from build123d import *
from OCP.BRepFilletAPI import BRepFilletAPI_MakeChamfer
from build123d.topology import SkipClean

# Parameters (mm, degrees)
SKETCH2_R           = 40
SKETCH2_R_2         = 20
BOSS_EXTRUDE1_DEPTH = 8
BOSS_EXTRUDE2_DEPTH = 12
SKETCH4_R           = 7.5
CUT_EXTRUDE1_DEPTH  = 10
SKETCH5_R           = 4
CUT_EXTRUDE2_DEPTH  = 29
BOSS_EXTRUDE3_DEPTH = 8
CHAMFER3_SIZE       = 8
CHAMFER3_SIZE_2     = 19.800694827
BOSS_EXTRUDE4_DEPTH = 12
FILLET1_R           = 6
CUT_EXTRUDE3_DEPTH  = 6
SKETCH9_R           = 4.2
CUT_EXTRUDE4_DEPTH  = 6
CUT_EXTRUDE5_START  = -22
CUT_EXTRUDE5_DEPTH  = 22


with BuildPart() as part:
    # Sketch2 → Boss-Extrude1 (new body)
    with BuildSketch(Plane.XY):
        Circle(SKETCH2_R)
        Circle(SKETCH2_R_2, mode=Mode.SUBTRACT)
    extrude(amount=BOSS_EXTRUDE1_DEPTH)

    # Sketch3 → Boss-Extrude2 (add)
    with BuildSketch(Plane(origin=(0, 0, 0), x_dir=(-1, 0, 0), z_dir=(0, 0, -1))):
        with BuildLine():
            Line((105, -25), (105, 25))
            Line((105, 25), (20.894189842, 56.244402662))
            ThreePointArc((20.894189842, 56.244402662), (-60, 0), (20.894189842, -56.244402662))
            Line((20.894189842, -56.244402662), (105, -25))
        make_face()
    extrude(amount=BOSS_EXTRUDE2_DEPTH)

    # Sketch4 → Cut-Extrude1 (cut)
    with BuildSketch(Plane(origin=(0, 0, -12), x_dir=(-1, 0, 0), z_dir=(0, 0, -1))):
        with Locations((0, 30)):
            Circle(SKETCH4_R)
        with Locations((30, 0)):
            Circle(SKETCH4_R)
        with Locations((0, -30)):
            Circle(SKETCH4_R)
        with Locations((-30, 0)):
            Circle(SKETCH4_R)
    extrude(amount=-CUT_EXTRUDE1_DEPTH, mode=Mode.SUBTRACT)

    # Sketch5 → Cut-Extrude2 (cut)
    with BuildSketch(Plane(origin=(0, 0, -2), x_dir=(-1, 0, 0), z_dir=(0, 0, -1))):
        with Locations((30, 0)):
            Circle(SKETCH5_R)
        with Locations((0, -30)):
            Circle(SKETCH5_R)
        with Locations((-30, 0)):
            Circle(SKETCH5_R)
        with Locations((0, 30)):
            Circle(SKETCH5_R)
    extrude(amount=-CUT_EXTRUDE2_DEPTH, mode=Mode.SUBTRACT)

    # Sketch6 → Boss-Extrude3 (add)
    with SkipClean():  # the faces are left unmerged after this step: merging them gives an invalid solid
        with BuildSketch(Plane.XY):
            with BuildLine():
                Line((39.290584114, -7.5), (59.529404499, -7.5))
                ThreePointArc((59.529404499, -7.5), (60, 0), (59.529404499, 7.5))
                Line((59.529404499, 7.5), (39.290584114, 7.5))
                ThreePointArc((39.290584114, 7.5), (40, 0), (39.290584114, -7.5))
            make_face()
            with BuildLine():
                Line((-7.5, 39.290584114), (-7.5, 59.529404499))
                ThreePointArc((-7.5, 59.529404499), (0, 60), (7.5, 59.529404499))
                Line((7.5, 59.529404499), (7.5, 39.290584114))
                ThreePointArc((7.5, 39.290584114), (0, 40), (-7.5, 39.290584114))
            make_face()
            with BuildLine():
                Line((-7.5, -39.290584114), (-7.5, -59.529404499))
                ThreePointArc((-7.5, -59.529404499), (0, -60), (7.5, -59.529404499))
                Line((7.5, -59.529404499), (7.5, -39.290584114))
                ThreePointArc((7.5, -39.290584114), (0, -40), (-7.5, -39.290584114))
            make_face()
            with BuildLine():
                Line((-39.290584114, 7.5), (-59.529404499, 7.5))
                ThreePointArc((-59.529404499, 7.5), (-60, 0), (-59.529404499, -7.5))
                Line((-59.529404499, -7.5), (-39.290584114, -7.5))
                ThreePointArc((-39.290584114, -7.5), (-40, 0), (-39.290584114, 7.5))
            make_face()
        extrude(amount=BOSS_EXTRUDE3_DEPTH)

    # Chamfer3
    chamfer3_edges_1 = [part.edges().sort_by_distance(p)[0] for p in [
        (0, 60, 8),
    ]]
    chamfer3_side_1 = [part.faces().sort_by_distance(p)[0] for p in [
        (0, 60, 7.84),
    ]]
    chamfer3_edges_2 = [part.edges().sort_by_distance(p)[0] for p in [
        (60, 0, 8),
    ]]
    chamfer3_side_2 = [part.faces().sort_by_distance(p)[0] for p in [
        (60, 0, 7.84),
    ]]
    chamfer3_edges_3 = [part.edges().sort_by_distance(p)[0] for p in [
        (-60, 0, 8),
    ]]
    chamfer3_side_3 = [part.faces().sort_by_distance(p)[0] for p in [
        (-60, 0, 7.84),
    ]]
    chamfer3_edges_4 = [part.edges().sort_by_distance(p)[0] for p in [
        (0, -60, 8),
    ]]
    chamfer3_side_4 = [part.faces().sort_by_distance(p)[0] for p in [
        (0, -60, 7.84),
    ]]
    chamfer3 = BRepFilletAPI_MakeChamfer(part.part.solid().wrapped)
    for e in chamfer3_edges_1:
        chamfer3.Add(CHAMFER3_SIZE - 0.0001, CHAMFER3_SIZE_2 - 0.0001, e.wrapped, chamfer3_side_1[0].wrapped)
    for e in chamfer3_edges_2:
        chamfer3.Add(CHAMFER3_SIZE - 0.0001, CHAMFER3_SIZE_2 - 0.0001, e.wrapped, chamfer3_side_2[0].wrapped)
    for e in chamfer3_edges_3:
        chamfer3.Add(CHAMFER3_SIZE - 0.0001, CHAMFER3_SIZE_2 - 0.0001, e.wrapped, chamfer3_side_3[0].wrapped)
    for e in chamfer3_edges_4:
        chamfer3.Add(CHAMFER3_SIZE - 0.0001, CHAMFER3_SIZE_2 - 0.0001, e.wrapped, chamfer3_side_4[0].wrapped)
    add(Compound.cast(chamfer3.Shape()), mode=Mode.REPLACE)  # a hair under: the kernel refuses the full size

    # Sketch7 → Boss-Extrude4 (add)
    with BuildSketch(Plane(origin=(0, 0, -12), x_dir=(-1, 0, 0), z_dir=(0, 0, -1))):
        with BuildLine():
            Line((115, 12.5), (105, 12.5))
            Line((105, 12.5), (105, -12.5))
            Line((105, -12.5), (115, -12.5))
            ThreePointArc((115, -12.5), (127.5, 0), (115, 12.5))
        make_face()
    extrude(amount=-BOSS_EXTRUDE4_DEPTH)

    # Fillet1
    fillet1_edges = [part.edges().sort_by_distance(p)[0] for p in [
        (-105, -25, -6),
        (-105, 25, -6),
        (-105, -12.5, -6),
        (-105, 12.5, -6),
    ]]
    fillet(fillet1_edges, radius=FILLET1_R)

    # Sketch8 → Cut-Extrude3 (cut)
    with SkipClean():  # the faces are left unmerged after this step: merging them gives an invalid solid
        with BuildSketch(Plane(origin=(0, 0, -12), x_dir=(-1, 0, 0), z_dir=(0, 0, -1))):
            Polygon((118.778590974, 6.485027647), (111.2730968, 6.514869597), (107.494505826, 0.02984195), (111.221409026, -6.485027647), (118.7269032, -6.514869597), (122.505494174, -0.02984195), align=None)
        extrude(amount=-CUT_EXTRUDE3_DEPTH, mode=Mode.SUBTRACT)

    # Sketch9 → Cut-Extrude4 (cut)
    with SkipClean():  # the faces are left unmerged after this step: merging them gives an invalid solid
        with BuildSketch(Plane(origin=(0, 0, -6), x_dir=(-1, 0, 0), z_dir=(0, 0, -1))):
            with Locations((115, 0)):
                Circle(SKETCH9_R)
        extrude(amount=-CUT_EXTRUDE4_DEPTH, mode=Mode.SUBTRACT)

    # Sketch10 → Cut-Extrude5 (cut)
    with SkipClean():  # the faces are left unmerged after this step: merging them gives an invalid solid
        with BuildSketch(Plane.XY.offset(CUT_EXTRUDE5_START)):
            with BuildLine():
                Line((-58.46152581, -13.5), (-93, -13.5))
                Line((-93, -13.5), (-93, -20.923688206))
                Line((-93, -20.923688206), (-46.167935821, -38.321295672))
                ThreePointArc((-46.167935821, -38.321295672), (-53.766674065, -26.62977206), (-58.46152581, -13.5))
            make_face()
            with BuildLine():
                Line((-93, 20.923688206), (-46.167935821, 38.321295672))
                ThreePointArc((-46.167935821, 38.321295672), (-53.766674065, 26.62977206), (-58.46152581, 13.5))
                Line((-58.46152581, 13.5), (-93, 13.5))
                Line((-93, 13.5), (-93, 20.923688206))
            make_face()
        extrude(amount=CUT_EXTRUDE5_DEPTH, mode=Mode.SUBTRACT)


solid = part.part
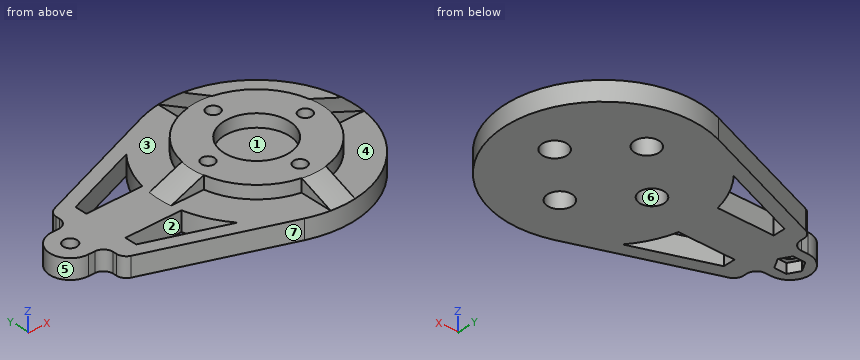
Geometry: final body of the model. Coordinates: model frame, mm. Face numbers are marked on the shaded views. A direction names the side the tool comes from. Round coordinates to 2 decimals unless told otherwise and drop trailing zeros. Loops run counter-clockwise (first coordinate to the right, second up) from the corner with the lowest first, then second, coordinate; pieces in that order, holes last.
Q1. Pull-direction query (Y, two-part tool) for the marked faces 5, 6 and 7; classes: released by +Y, released by -Y, zero draft, split by the parting line, or undercut.
Q2. Pin query (flat end, axial travel): P1, Ø6.5, axis at x = -48, z = 3.5, coming from the +Y side; P2, Ø5, axis at x = -94.5, y = 14.5, coming from the +Z side; P3, Ø9, axis at x = -53.5, z = 3, coming from the -Y side; P4, Ø7, axis at x = 0, y = -30, coming from the +Z side. Return the tip coordinate at first contact, or that it passes through.
Q3. Section A-A on x = 0. Return loops of the section in (y, z).
Q4. Section D-D on x = -30. Return loops of the section in (y, z).
Q5. Access query for the marked faces 1, 2, 3 and 4. Directions: +Z, -Z, +X, -X, +Y, -Y. A direction counts if a zero-diameter tool reaches every point of the face in a straight line with its end or side. Return the directions, or none.
Q6. Material intervals for L1, parallel to Y at x = -30, z = 0.75; L2, parallel to Y at x = 0, z = 3.5; L3, parallel to Y at x = 3, z = -0.25, sorted ascending.
Q7. Section C-C on y = -30. Return loops of the section in (x, z), plus the area to 3 significant figures.
Q8. Section B-B on z = 2.25. Return loops of the section in (x, y).
Evaluation:
1. face 5: split by the parting line
1. face 6: undercut
1. face 7: released by -Y
2. P1: stops at y = 7.5
2. P2: stops at z = 0
2. P3: stops at y = -45.38
2. P4: passes through
3. outline: (-60, -12) - (-37.5, -12) - (-37.5, -2) - (-34, -2) - (-34, 8) - (-40.2, 8) - (-60, 0) - close; (-26, -2) - (-22.5, -2) - (-22.5, -12) - (22.5, -12) - (22.5, -2) - (26, -2) - (26, 8) - (20, 8) - (20, 0) - (-20, 0) - (-20, 8) - (-26, 8) - close; (34, -2) - (37.5, -2) - (37.5, -12) - (60, -12) - (60, 0) - (40.2, 8) - (34, 8) - close
4. outline: (-52.86, -12) - (-7.5, -12) - (-7.5, -2) - (-4, -2) - (-4, 8) - (-26.46, 8) - (-26.46, 0) - (-52.86, 0) - close; (4, -2) - (7.5, -2) - (7.5, -12) - (52.86, -12) - (52.86, 0) - (26.46, 0) - (26.46, 8) - (4, 8) - close
5. face 1: +Z
5. face 2: +Z, -Z
5. face 3: +Z, -X
5. face 4: +Z, +X, -Y
6. L1: y = -26.46 to -4, 4 to 26.46
6. L2: y = -51.34 to -34, -26 to -20, 20 to 26, 34 to 51.34
6. L3: y = -59.92 to -32.65, -27.35 to 27.35, 32.65 to 59.92
7. outline: (-91.54, -12) - (-68.57, -12) - (-68.57, 0) - (-91.54, 0) - close; (-51.96, -12) - (-7.5, -12) - (-7.5, -2) - (-4, -2) - (-4, 8) - (-26.46, 8) - (-26.46, 0) - (-51.96, 0) - close; (4, -2) - (7.5, -2) - (7.5, -12) - (51.96, -12) - (51.96, 0) - (26.46, 0) - (26.46, 8) - (4, 8) - close
7. area: 1,720 mm2
8. outline: (-53.91, -7.5) - (-39.29, -7.5) arc R40 ccw to (-7.5, -39.29) - (-7.5, -53.91) arc R54.43 ccw to (7.5, -53.91) - (7.5, -39.29) arc R40 ccw to (39.29, -7.5) - (53.91, -7.5) arc R54.43 ccw to (53.91, 7.5) - (39.29, 7.5) arc R40 ccw to (7.5, 39.29) - (7.5, 53.91) arc R54.43 ccw to (-7.5, 53.91) - (-7.5, 39.29) arc R40 ccw to (-39.29, 7.5) - (-53.91, 7.5) arc R54.43 ccw to start; hole circle Ø8 at (-30, 0); hole circle Ø40 at (0, 0); hole circle Ø8 at (0, -30); hole circle Ø8 at (0, 30); hole circle Ø8 at (30, 0)
